Build history of the part. All positions in model axes, mm. Round coordinates to 2 decimals unless told otherwise and drop trailing zeros. Loops run counter-clockwise (first coordinate to the right, second up) from the corner with the lowest first, then second, coordinate; pieces in that order, holes last.
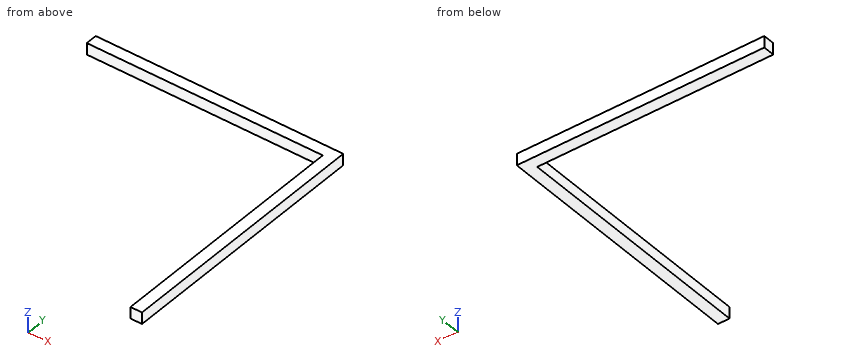
from build123d import *

# Parameters (mm, degrees)
F0_W     = 20
F0_H     = 20
F1_DEPTH = 450
F2_W     = 20
F2_H     = 20
F3_DEPTH = 410


with BuildPart() as f1:
    # F0 (on Front) → F1 (new body)
    with BuildSketch(Plane.XZ):
        with Locations((10, 10)):
            Rectangle(F0_W, F0_H)
    extrude(amount=F1_DEPTH)

    # F2 (on Right) → F3 (join)
    with BuildSketch(Plane.YZ):
        with Locations((-10, 10)):
            Rectangle(F2_W, F2_H)
    extrude(amount=-F3_DEPTH)


solid = f1.part
(1) Slice it at A-A on z = 12. List the corners of the cut face in (x, y), plus the area to 3 significant figures.
Responses:
outline: (-410, -20) - (0, -20) - (0, -450) - (20, -450) - (20, 0) - (-410, 0) - close
area: 17,200 mm2
(2) Pin check, flat tips, straight feed: P1, Ø10, axis at y = -143.5, z = 8, coming from the -X side; P2, Ø1.5, axis at x = -355.5, z = 15, coming from the -Y side. Stop position of each tip, or through.
Responses:
P1: stops at x = 0
P2: stops at y = -20
(3) Slice it at C-C on x = -313. List the corners of the cut face in (y, z).
Responses:
outline: (-20, 0) - (0, 0) - (0, 20) - (-20, 20) - close
(4) Probe line 1 (Y direction, x = -154, z = 1.5); line 2 (X direction, y = -335, z = 5.75). List the from-to ranges inside material, lowest first.
Responses:
line 1: y = -20 to 0
line 2: x = 0 to 20
(5) Slice it at B-B on y = -390. List the corners of the cut face in (x, z).
Responses:
outline: (0, 0) - (20, 0) - (20, 20) - (0, 20) - close
